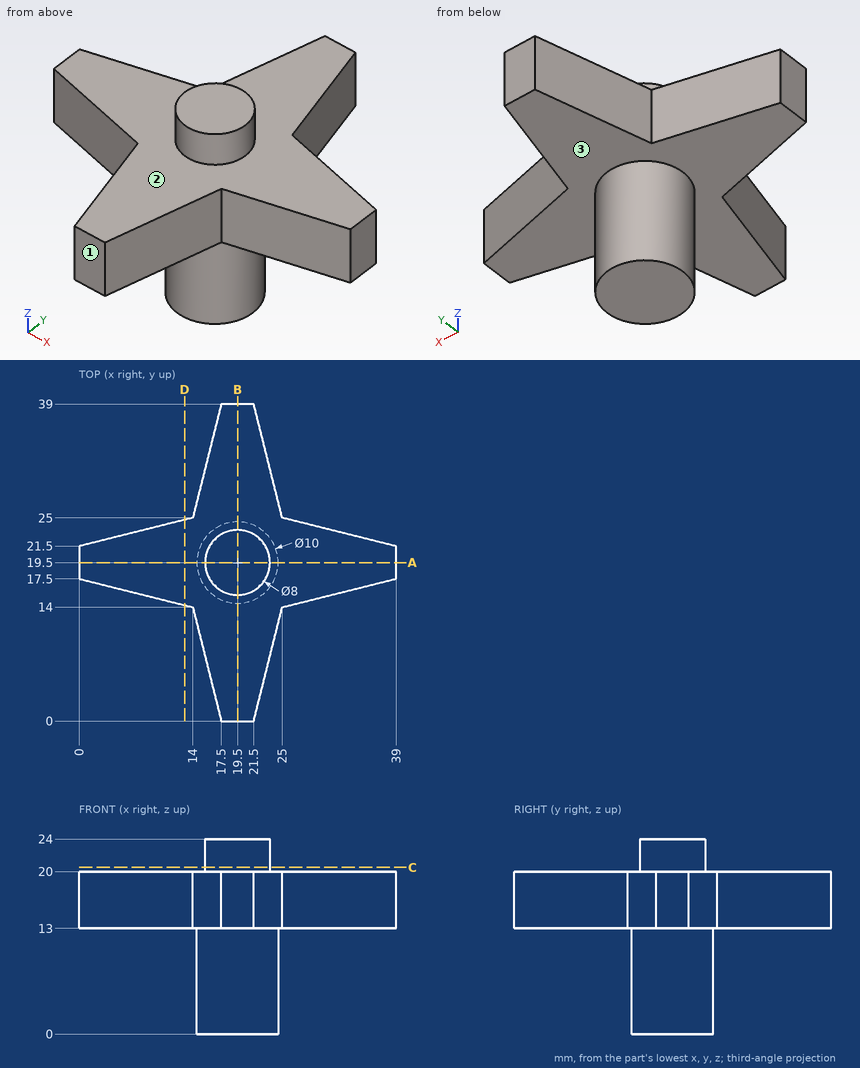
Part print with two shaded views. Sizes in mm from the minimum x, y, z corner. A direction names the side the tool comes from. Give positions to 0.01 mm unless a question says otherwise; leave off trailing zeros. Order: outer loops, then holes, each group sorted by start corner. A loop starts at its lowest first (then second) coordinate and runs counter-clockwise, first axis right, second up.
1) Saw through at C-C, the plane z = 20.5. Write the cut outline in (x, y), then the cut area to 3 significant figures.
2) Saw through at D-D, the plane x = 13. Write the cut outline in (y, z), then the cut area to 3 significant figures.
3) 3-axis set-ups, long thin cutter, end or side, ignore diameter. For the marked faces 1, 2 and 3: which of +Z, -Z, +X, -X, +Y, -Y reach the whole face in a straight line?
4) Saw through at A-A, the plane y = 19.5. Write the cut outline in (x, z), then the cut area to 3 significant figures.
5) Wall check: probe 1 along Z at (x, y) = (16, 9); probe 2 along X at (y, z) = (15.5, 3.25); probe 3 along X at (y, z) = (21.5, 8.5). Give the ranges that are in metal, low to high.
6) Pin check, flat tips, straight feed: pin 1 (8 mm diameter, centred on y = 14.5, z = 2.5, fed in from +X); pin 2 (5 mm diameter, centred on x = 31.5, y = 20.5, fed in from +Z); pin 3 (1 mm diameter, centred on x = 20, y = 32.5, fed in from -Z). Stop position of each tip, or through.
Computed:
1. outline: circle Ø8 at (19.5, 19.5)
1. area: 50.3 mm2
2. outline: (14.25, 13) - (24.75, 13) - (24.75, 20) - (14.25, 20) - close
2. area: 73.5 mm2
3. face 1: +Z, -Z, +X, -X, -Y
3. face 2: +Z
3. face 3: -Z
4. outline: (0, 13) - (14.5, 13) - (14.5, 0) - (24.5, 0) - (24.5, 13) - (39, 13) - (39, 20) - (23.5, 20) - (23.5, 24) - (15.5, 24) - (15.5, 20) - (0, 20) - close
4. area: 435 mm2
5. probe 1: z = 13 to 20
5. probe 2: x = 16.5 to 22.5
5. probe 3: x = 14.92 to 24.08
6. pin 1: stops at x = 24.4
6. pin 2: stops at z = 20
6. pin 3: stops at z = 13
